from build123d import *

# Parameters (mm, degrees)
F0_W     = 2500
F0_H     = 25
F0_R     = 1.5
F1_DEPTH = 3
F2_DEPTH = 25


with BuildPart() as f1:
    # F0 (on Front) → F1 (new body)
    with BuildSketch(Plane.XZ):
        with Locations((205.786598, 12.211518)):
            Rectangle(F0_W, F0_H)
        with Locations((-1031.713402, 12.211518)):
            Circle(F0_R, mode=Mode.SUBTRACT)
        with Locations((-911.713402, 12.211518)):
            Circle(F0_R, mode=Mode.SUBTRACT)
        with Locations((-791.713402, 12.211518)):
            Circle(F0_R, mode=Mode.SUBTRACT)
        with Locations((-671.713402, 12.211518)):
            Circle(F0_R, mode=Mode.SUBTRACT)
        with Locations((-551.713402, 12.211518)):
            Circle(F0_R, mode=Mode.SUBTRACT)
        with Locations((-431.713402, 12.211518)):
            Circle(F0_R, mode=Mode.SUBTRACT)
        with Locations((-311.713402, 12.211518)):
            Circle(F0_R, mode=Mode.SUBTRACT)
        with Locations((-191.713402, 12.211518)):
            Circle(F0_R, mode=Mode.SUBTRACT)
        with Locations((-71.713402, 12.211518)):
            Circle(F0_R, mode=Mode.SUBTRACT)
        with Locations((48.286598, 12.211518)):
            Circle(F0_R, mode=Mode.SUBTRACT)
    extrude(amount=F1_DEPTH)

    # F0 (on Front) → F2 (join)
    with BuildSketch(Plane.XZ):
        with Locations((-1031.713402, 12.211518)):
            Circle(F0_R)
        with Locations((-911.713402, 12.211518)):
            Circle(F0_R)
        with Locations((-791.713402, 12.211518)):
            Circle(F0_R)
        with Locations((-671.713402, 12.211518)):
            Circle(F0_R)
        with Locations((-551.713402, 12.211518)):
            Circle(F0_R)
        with Locations((-431.713402, 12.211518)):
            Circle(F0_R)
        with Locations((-311.713402, 12.211518)):
            Circle(F0_R)
        with Locations((-191.713402, 12.211518)):
            Circle(F0_R)
        with Locations((-71.713402, 12.211518)):
            Circle(F0_R)
        with Locations((48.286598, 12.211518)):
            Circle(F0_R)
    extrude(amount=F2_DEPTH)


solid = f1.part
Design review of the part built by this model. Coordinates are the model's own, in mm. Coordinates: 2 decimals unless noted, no trailing zeros. Order: outer loops, then holes, each group sorted by start corner. A loop starts at its lowest first (then second) coordinate and runs counter-clockwise, first axis right, second up. Notation, with made-up numbers: (69, -14) -> (81, -14) arc R7 cw to (81, -5) -> close; hole circle Ø3 at (-20.5, 84.25). An arc over 180 degrees is marked (long way). One line per item, written item: value.
1) We need section A-A, the plane y = -21. Count the separate pieces of the cut face and the enclosed holes in it, then the cut area to 3 significant figures.
Output values:
separate pieces: 10
enclosed holes: 0
area: 70.7 mm2
2) Clearance check with flat-ended pins moving along their axes: P1, Ø3, axis at x = 823.5, z = 8, coming from the -Y side; P2, Ø6, axis at x = 1123, z = 6.5, coming from the +Y side; P3, Ø5, axis at y = -17.5, z = 12, coming from the +X side; P4, Ø12, axis at y = -10, z = 5, coming from the +X side. State where each tip first meets the part, or that it passes through.
Output values:
P1: stops at y = -3
P2: stops at y = 0
P3: stops at x = 49.79
P4: stops at x = 49.17
3) We need section B-B, the plane x = -755. Give the boundary of the cut face in (y, z).
Output values:
outline: (-3, -0.29) -> (0, -0.29) -> (0, 24.71) -> (-3, 24.71) -> close
4) To check wall thickness, follow probe 1 along Y at (x, z) = (770, 7.75). State the ranges of the line that lie inside material, in increasing order. Write a range as [from, to].
Output values:
probe 1: y = [-3, 0]
